Source: CAD feature listing. Evaluate the final solid. Frame: model axes, mm. A direction names the side the tool comes from. Give positions to 0.01 mm unless a question says otherwise; leave off trailing zeros. Order: outer loops, then holes, each group sorted by start corner. A loop starts at its lowest first (then second) coordinate and runs counter-clockwise, first axis right, second up. Notation, with made-up numbers: M -39,49 L 11,49 A24 cw 11,79 Z; hole C 17.25,-4.5 d9. An arc over 180 degrees is marked long. Use CSV: the item, a comma, the result in double quotes. Start each with the question number.
1. Reachability of faces 1 (the flat face through (0, 23, -8)), 2 (the cylindrical face through (-1.42, 13.59, 0.81)) from +Z, -Z, +X, -X, +Y, -Y: full face, straight path, thin tool, end or side. Return the list, or none.
2. Section query C-C, the plane y = 17.25. State how many separate pieces and enclosed holes the cut face has, plus the area to 3 significant figures.
3. Section query B-B, the plane z = -12.75. Return the cut outline in (x, y).
4. Section query A-A, the plane x = 7. Return the cut outline in (y, z).
5. Pin query (flat end, axial travel): P1, Ø6, axis at y = 17.25, z = -12.75, coming from the -X side; P2, Ø10, axis at x = 1.5, y = 19.5, coming from the -Z side; P3, Ø2, axis at y = 15, z = -32, coming from the +X side. Return the tip coordinate at first contact, or that it passes through.
6. Line query: line 1 along Y through (x, z) = (-1.8, 0); line 2 along Y through (x, z) = (1.25, 0); line 3 along Z through (x, y) = (7.75, -2). Output: solid intervals per line, ascending. Write a range as [from, to].
7. Mould query, pull axis Z, two halves, no side actions, for faces 3 (the flat face through (6, -10, -14)), 4 (the cylindrical face through (6.177, -8.859, -36.547)), 5 (the flat face through (0, 15, -11)), 6 (the flat face through (0, -3, -27)). Classes: released by +Z, released by -Z, zero draft, split by the parting line, or undercut.
from build123d import *

# Parameters (mm, degrees)
SKETCH1_R           = 2.25
BOSS_EXTRUDE1_DEPTH = 2.6
BOSS_EXTRUDE3_START = -3
SKETCH3_R           = 3.75
BOSS_EXTRUDE3_DEPTH = 3
CHAMFER2_SIZE       = 0.3
CHAMFER3_SIZE       = 0.5
SKETCH4_R           = 2.25
BOSS_EXTRUDE4_DEPTH = 12.5


with BuildPart() as part:
    # Sketch1 → Boss-Extrude1 (new body)
    with BuildSketch(Plane(origin=(0, 0, 0), x_dir=(0, 0, -1), z_dir=(1, 0, 0))):
        with BuildLine():
            Line((-6, -10), (33.75, -10))
            ThreePointArc((33.75, -10), (36.578427125, -8.828427125), (37.75, -6))
            Line((37.75, -6), (37.75, 6))
            ThreePointArc((37.75, 6), (37.496577662, 7.401126626), (36.768422089, 8.62471486))
            Line((36.768422089, 8.62471486), (25.464074263, 21.62471486))
            ThreePointArc((25.464074263, 21.62471486), (24.104136506, 22.63997661), (22.445652174, 23))
            Line((22.445652174, 23), (-6, 23))
            ThreePointArc((-6, 23), (-8.828427125, 21.828427125), (-10, 19))
            Line((-10, 19), (-10, -6))
            ThreePointArc((-10, -6), (-8.828427125, -8.828427125), (-6, -10))
        make_face()
        with Locations((27.75, 0)):
            Circle(SKETCH1_R, mode=Mode.SUBTRACT)
        with Locations((0, 17.25)):
            Circle(SKETCH1_R, mode=Mode.SUBTRACT)
        Circle(SKETCH1_R, mode=Mode.SUBTRACT)
        with Locations((12.75, 17.25)):
            Circle(SKETCH1_R, mode=Mode.SUBTRACT)
    extrude(amount=BOSS_EXTRUDE1_DEPTH)

    # Sketch3 → Boss-Extrude3 (add)
    with BuildSketch(Plane(origin=(0, 0, 0), x_dir=(0, 0, -1), z_dir=(1, 0, 0)).offset(BOSS_EXTRUDE3_START)):
        with BuildLine():
            Line((-6, -10), (33.75, -10))
            ThreePointArc((33.75, -10), (36.578427125, -8.828427125), (37.75, -6))
            Line((37.75, -6), (37.75, 6))
            ThreePointArc((37.75, 6), (37.496577662, 7.401126626), (36.768422089, 8.62471486))
            Line((36.768422089, 8.62471486), (25.464074263, 21.62471486))
            ThreePointArc((25.464074263, 21.62471486), (24.104136506, 22.63997661), (22.445652174, 23))
            Line((22.445652174, 23), (-6, 23))
            ThreePointArc((-6, 23), (-8.828427125, 21.828427125), (-10, 19))
            Line((-10, 19), (-10, -6))
            ThreePointArc((-10, -6), (-8.828427125, -8.828427125), (-6, -10))
        make_face()
        with Locations((27.75, 0)):
            Circle(SKETCH3_R, mode=Mode.SUBTRACT)
        Circle(SKETCH3_R, mode=Mode.SUBTRACT)
        with Locations((0, 17.25)):
            Circle(SKETCH3_R, mode=Mode.SUBTRACT)
        with Locations((12.75, 17.25)):
            Circle(SKETCH3_R, mode=Mode.SUBTRACT)
    extrude(amount=BOSS_EXTRUDE3_DEPTH)

    # Chamfer2
    chamfer2_edges = [part.edges().sort_by_distance(p)[0] for p in [
        (0, 0, -25.5),
        (0, 17.25, 2.25),
        (0, 0, 2.25),
        (0, 17.25, -10.5),
        (0, 0, -24),
        (0, 0, 3.75),
        (0, 17.25, 3.75),
        (0, 17.25, -9),
    ]]
    chamfer(chamfer2_edges, length=CHAMFER2_SIZE)

    # Chamfer3
    chamfer3_edges = [part.edges().sort_by_distance(p)[0] for p in [
        (-3, -8.828427125, 8.828427125),
        (-3, 6.5, 10),
        (-3, 21.828427125, 8.828427125),
        (-3, 23, -8.222826087),
        (-3, 22.63997661, -24.104136506),
        (-3, 15.12471486, -31.116248176),
        (-3, 7.401126626, -37.496577662),
        (-3, 0, -37.75),
        (-3, -8.828427125, -36.578427125),
        (-3, -10, -13.875),
        (-3, 17.25, -9),
        (-3, 17.25, 3.75),
        (-3, 0, 3.75),
        (-3, 0, -24),
    ]]
    chamfer(chamfer3_edges, length=CHAMFER3_SIZE)

    # Sketch4 → Boss-Extrude4 (add)
    with BuildSketch(Plane(origin=(2.6, 0, 0), x_dir=(0, 0, -1), z_dir=(1, 0, 0))):
        with BuildLine():
            Line((-6, -10), (33.75, -10))
            ThreePointArc((33.75, -10), (36.578427125, -8.828427125), (37.75, -6))
            Line((37.75, -6), (37.75, 6))
            ThreePointArc((37.75, 6), (36.578427125, 8.828427125), (33.75, 10))
            Line((33.75, 10), (-6, 10))
            ThreePointArc((-6, 10), (-8.828427125, 8.828427125), (-10, 6))
            Line((-10, 6), (-10, -6))
            ThreePointArc((-10, -6), (-8.828427125, -8.828427125), (-6, -10))
        make_face()
        Circle(SKETCH4_R, mode=Mode.SUBTRACT)
        with Locations((27.75, 0)):
            Circle(SKETCH4_R, mode=Mode.SUBTRACT)
    extrude(amount=BOSS_EXTRUDE4_DEPTH)


solid = part.part
Result set:
1,face 1,"+Z, -Z, +X, -X, +Y"
1,face 2,"-X"
2,separate pieces,"3"
2,enclosed holes,"0"
2,area,"151 mm2"
3,outline,"M -3,-9.5 L -2.5,-10 L 15.1,-10 L 15.1,10 L 2.6,10 L 2.6,15 L 0.3,15 L 0,14.7 L 0,13.8 L -0.3,13.5 L -2.5,13.5 L -3,13 Z; M -3,21.5 L -2.5,21 L -0.3,21 L 0,20.7 L 0,19.8 L 0.3,19.5 L 2.6,19.5 L 2.6,23 L -2.5,23 L -3,22.5 Z"
4,outline,"M -10,-33.75 A4 ccw -6,-37.75 L 6,-37.75 A4 ccw 10,-33.75 L 10,6 A4 ccw 6,10 L -6,10 A4 ccw -10,6 Z; hole C 0,-27.75 d4.5; hole C 0,0 d4.5"
5,P1,"x = 0"
5,P2,"z = -31.66"
5,P3,"x = 2.6"
6,line 1,"[-10, -3.75], [3.75, 13.5], [21, 23]"
6,line 2,"[-10, -2.25], [2.25, 15], [19.5, 23]"
6,line 3,"[-37.75, -28.78], [-26.72, -1.03], [1.03, 10]"
7,face 3,"zero draft"
7,face 4,"released by -Z"
7,face 5,"undercut"
7,face 6,"undercut"
